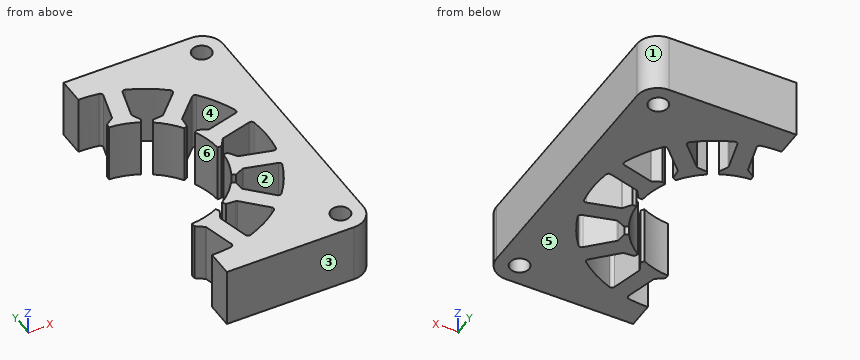
```python
from build123d import *

# Parameters (mm, degrees)
SKETCH1_W                              = 100
SKETCH1_H                              = 100
SKETCH1_R                              = 25.5
LAMINATION_EXTRUCTION_DEPTH            = 20
SLOT_CUT_DEPTH                         = 74.484692283
SLOT_FILLET_TOP_R                      = 1
SLOT_FILLET_BOTTOM_R                   = 0.5
SLOT_DUPLICATE_COUNT                   = 12
SLOT_FILLET_TOP_OF_SLOT_DUPLICATE_R    = 1
SLOT_FILLET_BOTTOM_OF_SLOT_DUPLICATE_R = 0.5
SKETCH3_R                              = 3.25
BOLT_HOLE_CUT_DEPTH                    = 74.484692283
CORNER_FILLET_R                        = 7
SKETCH4_W                              = 50
SKETCH4_H                              = 100
CUT_EXTRUDE1_DEPTH                     = 74.484692283


with BuildPart() as part:
    # Sketch1 → Lamination Extruction (new body)
    with BuildSketch(Plane.XY):
        Rectangle(SKETCH1_W, SKETCH1_H)
        Circle(SKETCH1_R, mode=Mode.SUBTRACT)
    extrude(amount=LAMINATION_EXTRUCTION_DEPTH)

    # Sketch2 → Slot Cut (cut, through all)
    with BuildSketch(Plane.XY.offset(20)):
        with BuildLine():
            Line((4.673479277, 28.779136449), (7.75, 40.260868098))
            ThreePointArc((7.75, 40.260868098), (0, 41), (-7.75, 40.260868098))
            Line((-7.75, 40.260868098), (-4.673479277, 28.779136449))
            Line((-4.673479277, 28.779136449), (-1.825, 26.784609787))
            Line((-1.825, 26.784609787), (-1.825, 25.434609787))
            ThreePointArc((-1.825, 25.434609787), (0, 25.5), (1.825, 25.434609787))
            Line((1.825, 25.434609787), (1.825, 26.784609787))
            Line((1.825, 26.784609787), (4.673479277, 28.779136449))
        make_face()
    slot_cut = extrude(amount=-SLOT_CUT_DEPTH, mode=Mode.SUBTRACT)

    # Slot Fillet Top
    slot_fillet_top_edges = [part.edges().sort_by_distance(p)[0] for p in [
        (-7.75, 40.260868098, 10),
        (7.75, 40.260868098, 10),
    ]]
    fillet(slot_fillet_top_edges, radius=SLOT_FILLET_TOP_R)

    # Slot Fillet Bottom
    slot_fillet_bottom_edges = [part.edges().sort_by_distance(p)[0] for p in [
        (4.673479277, 28.779136449, 10),
        (-4.673479277, 28.779136449, 10),
    ]]
    fillet(slot_fillet_bottom_edges, radius=SLOT_FILLET_BOTTOM_R)

    # Slot Duplicate: Slot Cut ×12 about axis
    slot_duplicate_axis = Axis((0, 0, 0), (0, 0, 1))
    for i in range(1, SLOT_DUPLICATE_COUNT):
        add(slot_cut.rotate(slot_duplicate_axis, i * 360 / SLOT_DUPLICATE_COUNT), mode=Mode.SUBTRACT)

    # Slot Fillet Top of Slot Duplicate
    slot_fillet_top_of_slot_duplicate_edges = [part.edges().sort_by_distance(p)[0] for p in [
        (-26.842130928, 30.991934551, 10),
        (-13.41873717, 38.741934551, 10),
        (-38.741934551, 13.41873717, 10),
        (-30.991934551, 26.842130928, 10),
        (-40.260868098, -7.75, 10),
        (-40.260868098, 7.75, 10),
        (-30.991934551, -26.842130928, 10),
        (-38.741934551, -13.41873717, 10),
        (-13.41873717, -38.741934551, 10),
        (-26.842130928, -30.991934551, 10),
        (7.75, -40.260868098, 10),
        (-7.75, -40.260868098, 10),
        (26.842130928, -30.991934551, 10),
        (13.41873717, -38.741934551, 10),
        (38.741934551, -13.41873717, 10),
        (30.991934551, -26.842130928, 10),
        (40.260868098, 7.75, 10),
        (40.260868098, -7.75, 10),
        (30.991934551, 26.842130928, 10),
        (38.741934551, 13.41873717, 10),
        (13.41873717, 38.741934551, 10),
        (26.842130928, 30.991934551, 10),
    ]]
    fillet(slot_fillet_top_of_slot_duplicate_edges, radius=SLOT_FILLET_TOP_OF_SLOT_DUPLICATE_R)

    # Slot Fillet Bottom of Slot Duplicate
    slot_fillet_bottom_of_slot_duplicate_edges = [part.edges().sort_by_distance(p)[0] for p in [
        (-10.342216447, 27.260202902, 10),
        (-18.436920002, 22.586723625, 10),
        (-22.586723625, 18.436920002, 10),
        (-27.260202902, 10.342216447, 10),
        (-28.779136449, 4.673479277, 10),
        (-28.779136449, -4.673479277, 10),
        (-27.260202902, -10.342216447, 10),
        (-22.586723625, -18.436920002, 10),
        (-18.436920002, -22.586723625, 10),
        (-10.342216447, -27.260202902, 10),
        (-4.673479277, -28.779136449, 10),
        (4.673479277, -28.779136449, 10),
        (10.342216447, -27.260202902, 10),
        (18.436920002, -22.586723625, 10),
        (22.586723625, -18.436920002, 10),
        (27.260202902, -10.342216447, 10),
        (28.779136449, -4.673479277, 10),
        (28.779136449, 4.673479277, 10),
        (27.260202902, 10.342216447, 10),
        (22.586723625, 18.436920002, 10),
        (18.436920002, 22.586723625, 10),
        (10.342216447, 27.260202902, 10),
    ]]
    fillet(slot_fillet_bottom_of_slot_duplicate_edges, radius=SLOT_FILLET_BOTTOM_OF_SLOT_DUPLICATE_R)

    # Sketch3 → Bolt Hole Cut (cut, through all)
    with BuildSketch(Plane.XY.offset(20)):
        with Locations((-42.5, 42.5)):
            Circle(SKETCH3_R)
        with Locations((42.5, 42.5)):
            Circle(SKETCH3_R)
        with Locations((42.5, -42.5)):
            Circle(SKETCH3_R)
        with Locations((-42.5, -42.5)):
            Circle(SKETCH3_R)
    extrude(amount=-BOLT_HOLE_CUT_DEPTH, mode=Mode.SUBTRACT)

    # Corner Fillet
    corner_fillet_edges = [part.edges().sort_by_distance(p)[0] for p in [
        (-50, 50, 10),
        (50, 50, 10),
        (50, -50, 10),
        (-50, -50, 10),
    ]]
    fillet(corner_fillet_edges, radius=CORNER_FILLET_R)

    # Sketch4 → Cut-Extrude1 (cut, through all)
    with BuildSketch(Plane.XY.offset(20)):
        with Locations((-25, 0)):
            Rectangle(SKETCH4_W, SKETCH4_H)
    extrude(amount=-CUT_EXTRUDE1_DEPTH, mode=Mode.SUBTRACT)


solid = part.part
```
Here's how the part is built. I have some questions about the finished solid (model axes, mm). Face numbers are marked on the shaded views. A direction names the side the tool comes from. Round coordinates to 2 decimals unless told otherwise and drop trailing zeros. Write each loop counter-clockwise with the first axis right and the second up, starting at its lowest first coordinate (ties: lowest second). Pieces come first, ordered by that corner, then holes.
Q1. Please list where these lines run through material, in increasing order: probe 1 along Y at (x, z) = (42.5, 14.5); probe 2 along Y at (x, z) = (34, 18); probe 3 along Y at (x, z) = (35, 18.25).
Q2. Will these pins go through, and if not, where does the flat tip stop? P1, Ø12, axis at y = -33, z = 14, coming from the -X side; P2, Ø6, axis at y = 9.5, z = 2.5, coming from the -X side; P3, Ø1.1, axis at y = -26, z = 10.5, coming from the -X side (3 decimals).
Q3. Which directions (+Z, -Z, +X, -X, +Y, -Y) give clear straight access to the entire face, cutting with the end or side of a thin tool? Please do the marked faces 4, 5 and 6.
Q4. If we section it at A-A on x = 42: Write out the boundary of the cut face in (y, z).
Q5. If we mould it in two halves opening along Y, with no side actions, what happens to the marked faces 1, 2 and 3? For each: +Y half, -Y half, draft (parallel to the pull), parting line (faces both ways), or undercut.
Q6. If we section it at B-B on y = 33: Write out the boundary of the cut face in (x, z), plus the area to 3 significant figures.
Q7. If we section it at C-C on z = 13.25: Give the number of separate pieces and of enclosed holes in the cut face, plus the area to 3 significant figures.
Answer below:
1. probe 1: y = -50 to -45.75, -39.25 to 39.25, 45.75 to 50
1. probe 2: y = -50 to -22.91, -12.15 to -6.07, 6.07 to 12.15, 22.91 to 50
1. probe 3: y = -50 to -21.35, -12.42 to -6.34, 6.34 to 12.42, 21.35 to 50
2. P1: stops at x = 2.13
2. P2: stops at x = 22.94
2. P3: stops at x = 1.825
3. face 4: +Z, -Z
3. face 5: -Z, +X, -X, +Y, -Y
3. face 6: +Z, -Z, -X
4. outline: (-50, 0) - (-45.71, 0) - (-45.71, 20) - (-50, 20) - close; (-39.29, 0) - (39.29, 0) - (39.29, 20) - (-39.29, 20) - close; (45.71, 0) - (50, 0) - (50, 20) - (45.71, 20) - close
5. face 1: +Y half
5. face 2: undercut
5. face 3: -Y half
6. outline: (5.8, 0) - (11.88, 0) - (11.88, 20) - (5.8, 20) - close; (24.33, 0) - (50, 0) - (50, 20) - (24.33, 20) - close
6. area: 635 mm2
7. separate pieces: 1
7. enclosed holes: 2
7. area: 2,890 mm2
